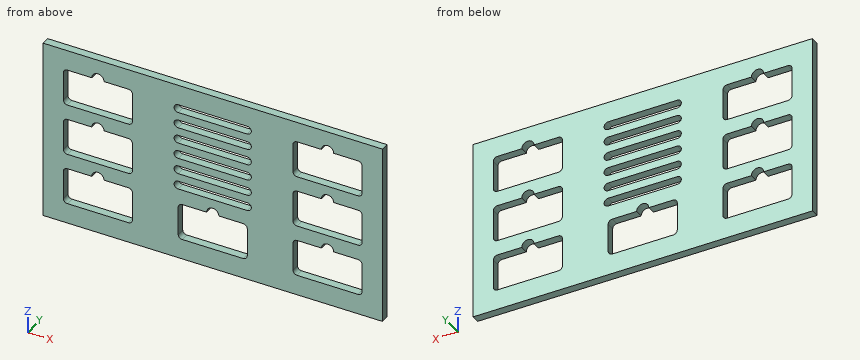
from build123d import *

# Parameters (mm, degrees)
SKETCH1_W           = 83.5
SKETCH1_H           = 44.4
BOSS_EXTRUDE1_DEPTH = 2


with BuildPart() as part:
    # Sketch1 → Boss-Extrude1 (new body)
    with BuildSketch(Plane(origin=(0, 0, 0), x_dir=(1, 0, 0), z_dir=(0, 1, 0))):
        with Locations((36.75, -17.2)):
            Rectangle(SKETCH1_W, SKETCH1_H)
        with BuildLine():
            Line((29.25, -9), (35.25, -9))
            ThreePointArc((35.25, -9), (36.75, -10.5), (38.25, -9))
            Line((38.25, -9), (44.25, -9))
            ThreePointArc((44.25, -9), (44.957106781, -8.707106781), (45.25, -8))
            Line((45.25, -8), (45.25, -1))
            ThreePointArc((45.25, -1), (44.957106781, -0.292893219), (44.25, 0))
            Line((44.25, 0), (29.25, 0))
            ThreePointArc((29.25, 0), (28.542893219, -0.292893219), (28.25, -1))
            Line((28.25, -1), (28.25, -8))
            ThreePointArc((28.25, -8), (28.542893219, -8.707106781), (29.25, -9))
        make_face(mode=Mode.SUBTRACT)
        with BuildLine():
            Line((1, 0), (16, 0))
            ThreePointArc((16, 0), (16.707106781, -0.292893219), (17, -1))
            Line((17, -1), (17, -8))
            ThreePointArc((17, -8), (16.707106781, -8.707106781), (16, -9))
            Line((16, -9), (10, -9))
            ThreePointArc((10, -9), (8.5, -10.5), (7, -9))
            Line((7, -9), (1, -9))
            ThreePointArc((1, -9), (0.292893219, -8.707106781), (0, -8))
            Line((0, -8), (0, -1))
            ThreePointArc((0, -1), (0.292893219, -0.292893219), (1, 0))
        make_face(mode=Mode.SUBTRACT)
        with BuildLine():
            Line((57.5, -9), (63.5, -9))
            ThreePointArc((63.5, -9), (65, -10.5), (66.5, -9))
            Line((66.5, -9), (72.5, -9))
            ThreePointArc((72.5, -9), (73.207106781, -8.707106781), (73.5, -8))
            Line((73.5, -8), (73.5, -1))
            ThreePointArc((73.5, -1), (73.207106781, -0.292893219), (72.5, 0))
            Line((72.5, 0), (57.5, 0))
            ThreePointArc((57.5, 0), (56.792893219, -0.292893219), (56.5, -1))
            Line((56.5, -1), (56.5, -8))
            ThreePointArc((56.5, -8), (56.792893219, -8.707106781), (57.5, -9))
        make_face(mode=Mode.SUBTRACT)
        with BuildLine():
            Line((57.5, -21.7), (63.5, -21.7))
            ThreePointArc((63.5, -21.7), (65, -23.2), (66.5, -21.7))
            Line((66.5, -21.7), (72.5, -21.7))
            ThreePointArc((72.5, -21.7), (73.207106781, -21.407106781), (73.5, -20.7))
            Line((73.5, -20.7), (73.5, -13.7))
            ThreePointArc((73.5, -13.7), (73.207106781, -12.992893219), (72.5, -12.7))
            Line((72.5, -12.7), (57.5, -12.7))
            ThreePointArc((57.5, -12.7), (56.792893219, -12.992893219), (56.5, -13.7))
            Line((56.5, -13.7), (56.5, -20.7))
            ThreePointArc((56.5, -20.7), (56.792893219, -21.407106781), (57.5, -21.7))
        make_face(mode=Mode.SUBTRACT)
        with BuildLine():
            Line((57.5, -34.4), (63.5, -34.4))
            ThreePointArc((63.5, -34.4), (65, -35.9), (66.5, -34.4))
            Line((66.5, -34.4), (72.5, -34.4))
            ThreePointArc((72.5, -34.4), (73.207106781, -34.107106781), (73.5, -33.4))
            Line((73.5, -33.4), (73.5, -26.4))
            ThreePointArc((73.5, -26.4), (73.207106781, -25.692893219), (72.5, -25.4))
            Line((72.5, -25.4), (57.5, -25.4))
            ThreePointArc((57.5, -25.4), (56.792893219, -25.692893219), (56.5, -26.4))
            Line((56.5, -26.4), (56.5, -33.4))
            ThreePointArc((56.5, -33.4), (56.792893219, -34.107106781), (57.5, -34.4))
        make_face(mode=Mode.SUBTRACT)
        with BuildLine():
            Line((1, -21.7), (7, -21.7))
            ThreePointArc((7, -21.7), (8.5, -23.2), (10, -21.7))
            Line((10, -21.7), (16, -21.7))
            ThreePointArc((16, -21.7), (16.707106781, -21.407106781), (17, -20.7))
            Line((17, -20.7), (17, -13.7))
            ThreePointArc((17, -13.7), (16.707106781, -12.992893219), (16, -12.7))
            Line((16, -12.7), (1, -12.7))
            ThreePointArc((1, -12.7), (0.292893219, -12.992893219), (0, -13.7))
            Line((0, -13.7), (0, -20.7))
            ThreePointArc((0, -20.7), (0.292893219, -21.407106781), (1, -21.7))
        make_face(mode=Mode.SUBTRACT)
        with BuildLine():
            Line((1, -34.4), (7, -34.4))
            ThreePointArc((7, -34.4), (8.5, -35.9), (10, -34.4))
            Line((10, -34.4), (16, -34.4))
            ThreePointArc((16, -34.4), (16.707106781, -34.107106781), (17, -33.4))
            Line((17, -33.4), (17, -26.4))
            ThreePointArc((17, -26.4), (16.707106781, -25.692893219), (16, -25.4))
            Line((16, -25.4), (1, -25.4))
            ThreePointArc((1, -25.4), (0.292893219, -25.692893219), (0, -26.4))
            Line((0, -26.4), (0, -33.4))
            ThreePointArc((0, -33.4), (0.292893219, -34.107106781), (1, -34.4))
        make_face(mode=Mode.SUBTRACT)
        with BuildLine():
            Line((28.25, -16.64), (45.25, -16.64))
            ThreePointArc((45.25, -16.64), (46.25, -17.64), (45.25, -18.64))
            Line((45.25, -18.64), (28.25, -18.64))
            ThreePointArc((28.25, -18.64), (27.25, -17.64), (28.25, -16.64))
        make_face(mode=Mode.SUBTRACT)
        with BuildLine():
            Line((28.25, -12.7), (45.25, -12.7))
            ThreePointArc((45.25, -12.7), (46.25, -13.7), (45.25, -14.7))
            Line((45.25, -14.7), (28.25, -14.7))
            ThreePointArc((28.25, -14.7), (27.25, -13.7), (28.25, -12.7))
        make_face(mode=Mode.SUBTRACT)
        with BuildLine():
            Line((28.25, -20.58), (45.25, -20.58))
            ThreePointArc((45.25, -20.58), (46.25, -21.58), (45.25, -22.58))
            Line((45.25, -22.58), (28.25, -22.58))
            ThreePointArc((28.25, -22.58), (27.25, -21.58), (28.25, -20.58))
        make_face(mode=Mode.SUBTRACT)
        with BuildLine():
            Line((28.25, -24.52), (45.25, -24.52))
            ThreePointArc((45.25, -24.52), (46.25, -25.52), (45.25, -26.52))
            Line((45.25, -26.52), (28.25, -26.52))
            ThreePointArc((28.25, -26.52), (27.25, -25.52), (28.25, -24.52))
        make_face(mode=Mode.SUBTRACT)
        with BuildLine():
            Line((28.25, -28.46), (45.25, -28.46))
            ThreePointArc((45.25, -28.46), (46.25, -29.46), (45.25, -30.46))
            Line((45.25, -30.46), (28.25, -30.46))
            ThreePointArc((28.25, -30.46), (27.25, -29.46), (28.25, -28.46))
        make_face(mode=Mode.SUBTRACT)
        with BuildLine():
            Line((28.25, -32.4), (45.25, -32.4))
            ThreePointArc((45.25, -32.4), (46.25, -33.4), (45.25, -34.4))
            Line((45.25, -34.4), (28.25, -34.4))
            ThreePointArc((28.25, -34.4), (27.25, -33.4), (28.25, -32.4))
        make_face(mode=Mode.SUBTRACT)
    extrude(amount=BOSS_EXTRUDE1_DEPTH)


solid = part.part
Could you check a few things on this model? Use its own coordinates, in mm. Coordinates: 2 decimals unless noted, no trailing zeros. Write each loop counter-clockwise with the first axis right and the second up, starting at its lowest first coordinate (ties: lowest second). Pieces come first, ordered by that corner, then holes. Notation, with made-up numbers: (2, 28) - (60, 28) arc R33 ccw to (60, 65) - close; hole circle Ø9 at (-39.75, 72.25). An arc over 180 degrees is marked (long way). Write item = value, one per line.
1) Suppose I cut it at B-B on z = 15.5. Please give me the cut outline in (x, y).
Result set:
outline = (-5, 0) - (0, 0) - (0, 2) - (-5, 2) - close; (17, 0) - (56.5, 0) - (56.5, 2) - (17, 2) - close; (73.5, 0) - (78.5, 0) - (78.5, 2) - (73.5, 2) - close
2) Please list where these lines run through material, in increasing order: line 1 (Z direction, x = 5.5, y = 0.4); line 2 (X direction, y = 1.7, z = 19.5); line 3 (X direction, y = 0.1, z = 1.5). Write a range as [from, to].
Result set:
line_1 = [-5, 0], [9, 12.7], [21.7, 25.4], [34.4, 39.4]
line_2 = [-5, 0], [17, 56.5], [73.5, 78.5]
line_3 = [-5, 0], [17, 28.25], [45.25, 56.5], [73.5, 78.5]
3) Suppose I cut it at C-C on x = 36.75. State how many separate pieces and enclosed holes the cut face has, plus the area to 3 significant figures.
Result set:
separate_pieces = 8
enclosed_holes = 0
area = 43.8 mm2
4) Suppose I cut it at A-A on x = 8.5. Please give me the cut outline in (y, z).
Result set:
outline = (0, -5) - (2, -5) - (2, 0) - (0, 0) - close; (0, 10.5) - (2, 10.5) - (2, 12.7) - (0, 12.7) - close; (0, 23.2) - (2, 23.2) - (2, 25.4) - (0, 25.4) - close; (0, 35.9) - (2, 35.9) - (2, 39.4) - (0, 39.4) - close
